Geometry check sheet. Reference: the model listing, model coordinates, mm. A direction names the side the tool comes from. Round coordinates to 2 decimals unless told otherwise and drop trailing zeros. Write each loop counter-clockwise with the first axis right and the second up, starting at its lowest first coordinate (ties: lowest second). Pieces come first, ordered by that corner, then holes. Notation, with made-up numbers: M 31.5,57 L 64.5,57 A19 cw 64.5,83 Z; hole C 55.25,23.25 d11. An arc over 180 degrees is marked long. Put each result on its own line as item: value. Start each with the question number.
(1) Section check A-A on z = 65. Record the cut outline in (x, y).
(2) Mould release check, pull along Z, two halves, no side actions. Record for faces 1 (the flat face through (-50, 0, 156.918)), 2 (the cylindrical face through (-23.644, 1.915, 125.381)), 3 (the flat face through (215.096, 15, 130)): pulls with the +Z half, pulls with the -Z half, needs draft (parallel to the pull), parting line crosses it, or undercut.
(3) Section check B-B on x = 64.5. Record the cut outline in (y, z), then the cut area to 3 significant figures.
(4) Section check C-C on z = 17. Record the cut outline in (x, y), then the cut area to 3 significant figures.
(5) Gauge pin test, flat ends, axial feed: pin 1 (4 mm diameter, centred on x = 218, z = 150, fed in from -Y); pin 2 (10 mm diameter, centred on x = 60, y = -11, fed in from +Z); pin 3 (17.5 mm diameter, centred on y = -3.5, z = 104.5, fed in from +X); pin 4 (1 mm diameter, centred on y = -9, z = 65.5, fed in from +X). Record the tip position at first contact, or that the pin passes through.
(6) Section check D-D on y = 0. Count the separate pieces of the cut face and the enclosed holes in it, then the cut area to 3 significant figures.
(7) Tool access check on faces 4 (the flat face through (203, 11, 79)), 5 (the flat face through (220.096, 0, 152)), 6 (the flat face through (-52.904, 0, 152)), 7 (the flat face through (85, -11, 13)). Record the directions out of +Z, -Z, +X, -X, +Y, -Y that give a thin tool (end or side, any length) a straight path to the whole face; none if there is none.
(8) Material ranges on probe 1 along X at (y, z) = (9, 59); probe 2 along Y at (x, z) = (-28, 8); probe 3 along Y at (x, z) = (214.6, 130), recorded low to high.
from build123d import *

# Parameters (mm, degrees)
SKETCH3_W           = 25
SKETCH3_H           = 25
SKETCH3_W_2         = 22
SKETCH3_H_2         = 22
BOSS_EXTRUDE1_DEPTH = 160
SKETCH4_W           = 25
SKETCH4_H           = 25
SKETCH4_W_2         = 22
SKETCH4_H_2         = 22
BOSS_EXTRUDE2_DEPTH = 106.5
SKETCH5_R           = 5
BOSS_EXTRUDE3_DEPTH = 10
SKETCH6_W           = 10
SKETCH6_H           = 12
CUT_EXTRUDE1_DEPTH  = 5
CUT_EXTRUDE2_START  = -25
SKETCH7_R           = 5
CUT_EXTRUDE2_DEPTH  = 25


with BuildPart() as part:
    # Sketch3 → Boss-Extrude1 (new body)
    with BuildSketch(Plane.XY):
        with Locations((-35.404260395, 0)):
            Rectangle(SKETCH3_W, SKETCH3_H)
        with Locations((-35.404260395, 0)):
            Rectangle(SKETCH3_W_2, SKETCH3_H_2, mode=Mode.SUBTRACT)
    boss_extrude1 = extrude(amount=BOSS_EXTRUDE1_DEPTH)

    # Sketch4 → Boss-Extrude2 (add)
    with BuildSketch(Plane(origin=(-22.904260395, 0, 0), x_dir=(0, 0, -1), z_dir=(1, 0, 0))):
        with Locations((-12.5, 0)):
            Rectangle(SKETCH4_W, SKETCH4_H)
        with Locations((-12.5, 0)):
            Rectangle(SKETCH4_W_2, SKETCH4_H_2, mode=Mode.SUBTRACT)
    boss_extrude2 = extrude(amount=BOSS_EXTRUDE2_DEPTH)

    # Sketch5 → Boss-Extrude3 (add)
    # profile 1 of 5: a face of its own
    with BuildSketch(Plane.ZY.offset(47.904260395)):
        with BuildLine():
            ThreePointArc((113.082291583, -6), (112.049822896, 0), (113.082291583, 6))
            Line((113.082291583, 6), (103.082291583, 6))
            Line((103.082291583, 6), (103.082291583, -6))
            Line((103.082291583, -6), (113.082291583, -6))
        make_face()
    # profile 2 of 5: a face of its own
    with BuildSketch(Plane.ZY.offset(47.904260395)):
        with BuildLine():
            ThreePointArc((147.950177104, 0), (147.69017694, 3.044092295), (146.917708417, 6))
            ThreePointArc((146.917708417, 6), (145.250430663, 9.467482384), (142.882502012, 12.5))
            Line((142.882502012, 12.5), (117.117497988, 12.5))
            ThreePointArc((117.117497988, 12.5), (114.749569337, 9.467482384), (113.082291583, 6))
            ThreePointArc((113.082291583, 6), (112.049822896, 0), (113.082291583, -6))
            ThreePointArc((113.082291583, -6), (114.749569337, -9.467482384), (117.117497988, -12.5))
            Line((117.117497988, -12.5), (142.882502012, -12.5))
            ThreePointArc((142.882502012, -12.5), (145.250430663, -9.467482384), (146.917708417, -6))
            ThreePointArc((146.917708417, -6), (147.69017694, -3.044092295), (147.950177104, 0))
        make_face()
        with Locations((130, 0)):
            Circle(SKETCH5_R, mode=Mode.SUBTRACT)
    # profile 3 of 5: a face of its own
    with BuildSketch(Plane.ZY.offset(47.904260395)):
        with BuildLine():
            Line((156.917708417, 6), (146.917708417, 6))
            ThreePointArc((146.917708417, 6), (147.69017694, 3.044092295), (147.950177104, 0))
            ThreePointArc((147.950177104, 0), (147.69017694, -3.044092295), (146.917708417, -6))
            Line((146.917708417, -6), (156.917708417, -6))
            Line((156.917708417, -6), (156.917708417, 6))
        make_face()
    # profile 4 of 5: a face of its own
    with BuildSketch(Plane.ZY.offset(47.904260395)):
        with BuildLine():
            Line((117.117497988, 12.5), (142.882502012, 12.5))
            ThreePointArc((142.882502012, 12.5), (130, 17.950177104), (117.117497988, 12.5))
        make_face()
    # profile 5 of 5: a face of its own
    with BuildSketch(Plane.ZY.offset(47.904260395)):
        with BuildLine():
            ThreePointArc((117.117497988, -12.5), (130, -17.950177104), (142.882502012, -12.5))
            Line((142.882502012, -12.5), (117.117497988, -12.5))
        make_face()
    boss_extrude3 = extrude(amount=BOSS_EXTRUDE3_DEPTH)

    # Sketch6 → Cut-Extrude1 (cut)
    with BuildSketch(Plane.ZY.offset(57.904260395)):
        with Locations((108.082291583, 0)):
            Rectangle(SKETCH6_W, SKETCH6_H)
        with Locations((151.917708417, 0)):
            Rectangle(SKETCH6_W, SKETCH6_H)
    cut_extrude1 = extrude(amount=-CUT_EXTRUDE1_DEPTH, mode=Mode.SUBTRACT)

    # Sketch7 → Cut-Extrude2 (cut)
    with BuildSketch(Plane.ZY.offset(47.904260395).offset(CUT_EXTRUDE2_START)):
        with Locations(Location((130, 0, 0), (0, 0, 180))):
            Circle(SKETCH7_R)
    cut_extrude2 = extrude(amount=CUT_EXTRUDE2_DEPTH, mode=Mode.SUBTRACT)

    # Mirror1: Boss-Extrude1, Boss-Extrude2, Boss-Extrude3, Cut-Extrude1, Cut-Extrude2 across plane
    add(boss_extrude1.mirror(Plane(origin=(83.595739605, 0, 0), x_dir=(0, 0, 1), z_dir=(1, 0, 0))))
    add(boss_extrude2.mirror(Plane(origin=(83.595739605, 0, 0), x_dir=(0, 0, 1), z_dir=(1, 0, 0))))
    add(boss_extrude3.mirror(Plane(origin=(83.595739605, 0, 0), x_dir=(0, 0, 1), z_dir=(1, 0, 0))))
    add(cut_extrude1.mirror(Plane(origin=(83.595739605, 0, 0), x_dir=(0, 0, 1), z_dir=(1, 0, 0))), mode=Mode.SUBTRACT)
    add(cut_extrude2.mirror(Plane(origin=(83.595739605, 0, 0), x_dir=(0, 0, 1), z_dir=(1, 0, 0))), mode=Mode.SUBTRACT)


solid = part.part
Answers follow:
1. outline: M -47.9,-12.5 L -22.9,-12.5 L -22.9,12.5 L -47.9,12.5 Z; M 190.1,-12.5 L 215.1,-12.5 L 215.1,12.5 L 190.1,12.5 Z; hole M -46.4,-11 L -24.4,-11 L -24.4,11 L -46.4,11 Z; hole M 191.6,-11 L 213.6,-11 L 213.6,11 L 191.6,11 Z
2. face 1: pulls with the +Z half
2. face 2: undercut
2. face 3: needs draft
3. outline: M -12.5,0 L 12.5,0 L 12.5,25 L -12.5,25 Z; hole M -11,1.5 L 11,1.5 L 11,23.5 L -11,23.5 Z
3. area: 141 mm^2
4. outline: M -47.9,-12.5 L 215.1,-12.5 L 215.1,12.5 L -47.9,12.5 Z; hole M -46.4,-11 L -24.4,-11 L -24.4,11 L -46.4,11 Z; hole M -22.9,-11 L 190.1,-11 L 190.1,11 L -22.9,11 Z; hole M 191.6,-11 L 213.6,-11 L 213.6,11 L 191.6,11 Z
4. area: 921 mm^2
5. pin 1: stops at y = -6
5. pin 2: stops at z = 25
5. pin 3: stops at x = 225.1
5. pin 4: stops at x = 215.1
6. separate pieces: 7
6. enclosed holes: 1
6. area: 2,220 mm^2
7. face 4: +Z, -Z
7. face 5: +Z, +X, +Y, -Y
7. face 6: +Z, -X, +Y, -Y
7. face 7: none
8. probe 1: x = -47.9 to -46.4, -24.4 to -22.9, 190.1 to 191.6, 213.6 to 215.1
8. probe 2: y = -12.5 to -11, 11 to 12.5
8. probe 3: y = -12.5 to -5, 5 to 12.5
